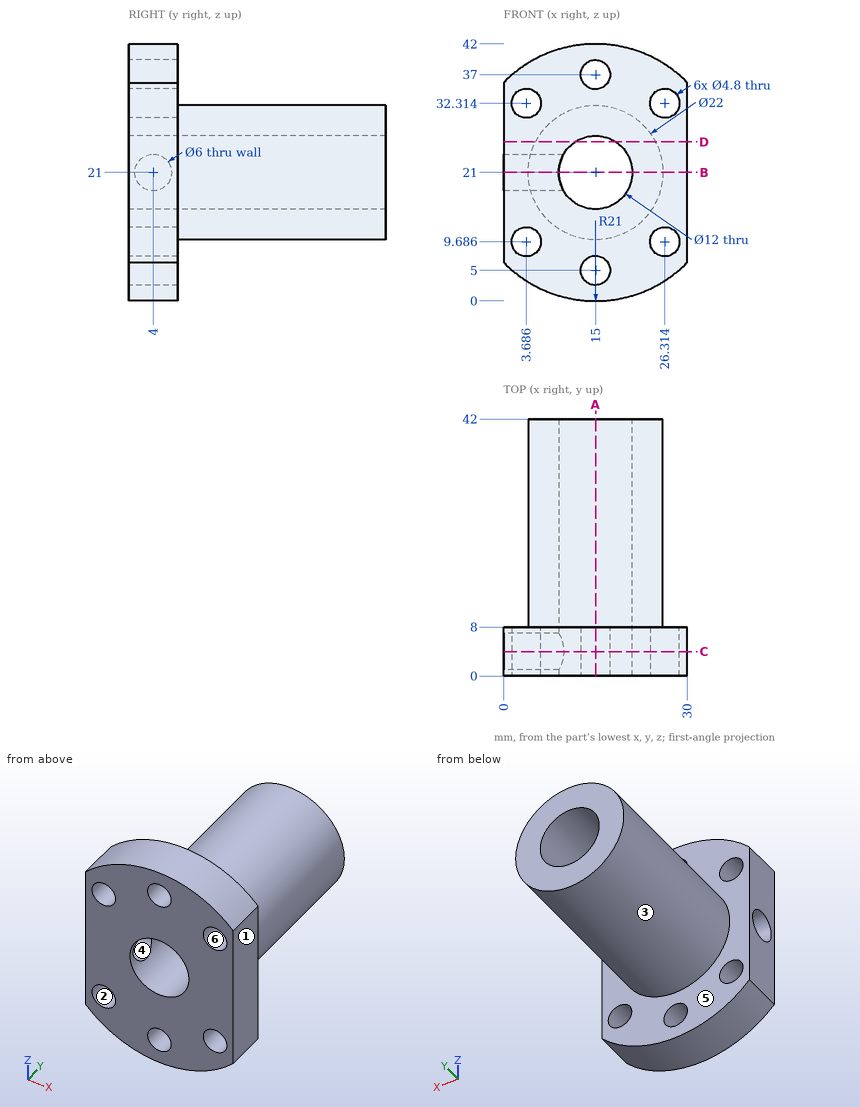
Can you work these out from the drawing? Everything is in mm from the part's minimum corner. A direction names the side the tool comes from. Give positions to 0.01 mm unless a question says otherwise; leave off trailing zeros. Order: outer loops, then holes, each group sorted by start corner. A loop starts at its lowest first (then second) coordinate and runs counter-clockwise, first axis right, second up. Notation, with made-up numbers: M 34,-12.5 L 56,-12.5 A29 cw 56,7.5 Z; hole C 74,72.25 d6. An arc over 180 degrees is marked long. Use a Markdown table: item, result. Add a question column.
Item 1: Will these pins go through, and if not, where does the flat tip stop? pin 1 (4 mm diameter, centred on x = 3.69, z = 32.31, fed in from +Y); pin 2 (10 mm diameter, centred on x = 17, y = 18.5, fed in from +Z); pin 3 (5 mm diameter, centred on y = 16.5, z = 26.5, fed in from -X); pin 4 (6 mm diameter, centred on x = 7.5, y = 7.5, fed in from -Z).
Item 2: We'd pull the mould along Z, two halves only. Please class the marked faces 1, 2, 3 and 4: +Z half, -Z half, draft (parallel to the pull), parting line (faces both ways), or undercut.
Item 3: Suppose I cut it at B-B (z = 21). List the corners of the cut face in (x, y) for me.
Item 4: For the marked faces 5 and 6, which set-ups out of +Z, -Z, +X, -X, +Y, -Y let a thin tool reach every point of the face, with its end or its side?
Item 5: If I drill on L1, parallel to X at y = 14, z = 21; L2, parallel to Z at x = 15, y = 30.5; L3, parallel to X at y = 5.5, z = 34.5 (1 decimal), over which ranges is the centre line in solid material (lowest first)? Write a range as [from, to].
Item 6: Suppose I cut it at C-C (y = 4). List the corners of the cut face in (x, z) for me.
Item 7: Suppose I cut it at A-A (x = 15). List the corners of the cut face in (y, z) for me.
Item 8: Suppose I cut it at D-D (z = 26). List the corners of the cut face in (x, y) for me.
Answer sheet:
| question | item | result |
|---|---|---|
| 1 | pin 1 | passes through |
| 1 | pin 2 | stops at z = 32 |
| 1 | pin 3 | stops at x = 4.42 |
| 1 | pin 4 | stops at z = 0.49 |
| 2 | face 1 | draft |
| 2 | face 2 | undercut |
| 2 | face 3 | parting line |
| 2 | face 4 | undercut |
| 3 | outline | M 0,0 L 9,0 L 9,1 L 0,1 Z; M 0,7 L 9,7 L 9,42 L 4,42 L 4,8 L 0,8 Z; M 21,0 L 30,0 L 30,8 L 26,8 L 26,42 L 21,42 Z |
| 4 | face 5 | +Y |
| 4 | face 6 | +Y, -Y |
| 5 | L1 | x = [4, 9], [21, 26] |
| 5 | L2 | z = [10, 15], [27, 32] |
| 5 | L3 | x = [0, 2.7], [4.7, 25.3], [27.3, 30] |
| 6 | outline | M 0,6.3 A21 ccw 30,6.3 L 30,35.7 A21 ccw 0,35.7 L 0,24 L 9.8,24 A6 cw long 9.8,18 L 0,18 Z; hole C 3.69,9.69 d4.8; hole C 3.69,32.31 d4.8; hole C 15,5 d4.8; hole C 15,37 d4.8; hole C 26.31,9.69 d4.8; hole C 26.31,32.31 d4.8 |
| 7 | outline | M 0,0 L 8,0 L 8,2.6 L 0,2.6 Z; M 0,7.4 L 8,7.4 L 8,10 L 42,10 L 42,15 L 0,15 Z; M 0,27 L 42,27 L 42,32 L 8,32 L 8,34.6 L 0,34.6 Z; M 0,39.4 L 8,39.4 L 8,42 L 0,42 Z |
| 8 | outline | M 0,0 L 11.68,0 L 11.68,42 L 5.2,42 L 5.2,8 L 0,8 Z; M 18.32,0 L 30,0 L 30,8 L 24.8,8 L 24.8,42 L 18.32,42 Z |
